Could you check a few things on this model? Use its own coordinates, in mm. Coordinates: 2 decimals unless noted, no trailing zeros. Write each loop counter-clockwise with the first axis right and the second up, starting at its lowest first coordinate (ties: lowest second). Pieces come first, ordered by that corner, then holes. Notation, with made-up numbers: M 48,81 L 99,81 A11 cw 99,93 Z; hole C 22.25,-25 d5. An arc over 180 degrees is marked long. Write item = value, one per line.
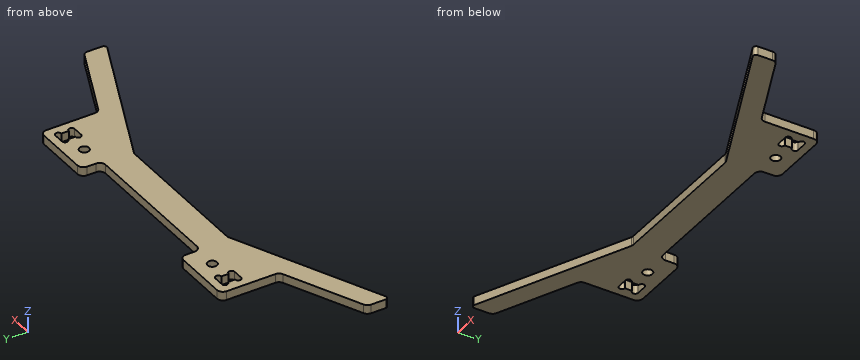
```python
from build123d import *

# Parameters (mm, degrees)
EXTRUDE_1_DEPTH     = 3
SKETCH_2_W          = 83.2
SKETCH_2_H          = 9
EXTRUDE_2_DEPTH     = 3
SKETCH_3_W          = 42.77133807
SKETCH_3_H          = 9.521513309
CUT_EXTRUDE_1_DEPTH = 3
EXTRUDE_3_DEPTH     = 3
CUT_EXTRUDE_2_DEPTH = 3
EXTRUDE_4_DEPTH     = 3
SKETCH_6_R          = 1.6
CUT_EXTRUDE_3_DEPTH = 3
SKETCH_8_W          = 53.2
SKETCH_8_H          = 7
CUT_EXTRUDE_4_DEPTH = 10
FILLET_2_R          = 2
FILLET_3_R          = 1


with BuildPart() as part:
    # 草图1 → 凸台-拉伸1 (new body)
    with BuildSketch(Plane.XY):
        Polygon((76.365250313, 0), (0, 34), (-76.365250313, 0), (-76.365250313, 6.567817671), (0, 40.567817671), (76.365250313, 6.567817671), align=None)
    extrude(amount=EXTRUDE_1_DEPTH)

    # 草图2 → 凸台-拉伸2 (add)
    with BuildSketch(Plane.XY.offset(3)):
        with Locations((0, 26.546304362)):
            Rectangle(SKETCH_2_W, SKETCH_2_H)
    extrude(amount=-EXTRUDE_2_DEPTH)

    # 草图3 → 切除-拉伸1 (cut)
    with BuildSketch(Plane.XY.offset(3)):
        with Locations((0, 35.807061017)):
            Rectangle(SKETCH_3_W, SKETCH_3_H)
    extrude(amount=-CUT_EXTRUDE_1_DEPTH, mode=Mode.SUBTRACT)

    # 草图4 → 凸台-拉伸3 (add)
    with BuildSketch(Plane.XY.offset(3)):
        Polygon((41.6, 31.046304362), (48.6, 31.046304362), (48.6, 18.929703565), (41.6, 22.046304362), align=None)
        Polygon((-41.6, 31.046304362), (-48.6, 31.046304362), (-48.6, 18.929703565), (-41.6, 22.046304362), align=None)
    extrude(amount=-EXTRUDE_3_DEPTH)

    # 草图5 → 切除-拉伸2 (cut)
    with BuildSketch(Plane.XY.offset(3)):
        with BuildLine():
            Line((-44.85, 28.296304362), (-41.35, 28.296304362))
            ThreePointArc((-41.35, 28.296304362), (-40.35, 27.296304362), (-41.35, 26.296304362))
            Line((-41.35, 26.296304362), (-41.35, 23.796304362))
            ThreePointArc((-41.35, 23.796304362), (-40.35, 22.796304362), (-41.35, 21.796304362))
            Line((-41.35, 21.796304362), (-44.85, 21.796304362))
            ThreePointArc((-44.85, 21.796304362), (-45.85, 22.796304362), (-44.85, 23.796304362))
            Line((-44.85, 23.796304362), (-44.85, 26.296304362))
            ThreePointArc((-44.85, 26.296304362), (-45.85, 27.296304362), (-44.85, 28.296304362))
        make_face()
        with BuildLine():
            Line((41.35, 26.296304362), (41.35, 23.796304362))
            ThreePointArc((41.35, 23.796304362), (40.35, 22.796304362), (41.35, 21.796304362))
            Line((41.35, 21.796304362), (44.85, 21.796304362))
            ThreePointArc((44.85, 21.796304362), (45.85, 22.796304362), (44.85, 23.796304362))
            Line((44.85, 23.796304362), (44.85, 26.296304362))
            ThreePointArc((44.85, 26.296304362), (45.85, 27.296304362), (44.85, 28.296304362))
            Line((44.85, 28.296304362), (41.35, 28.296304362))
            ThreePointArc((41.35, 28.296304362), (40.35, 27.296304362), (41.35, 26.296304362))
        make_face()
    extrude(amount=-CUT_EXTRUDE_2_DEPTH, mode=Mode.SUBTRACT)

    # 草图7 → 凸台-拉伸4 (add)
    with BuildSketch(Plane.XY.offset(3)):
        Polygon((26.848439987, 22.046304362), (76.365250313, 0), (76.365250313, -8.757090228), (25.147987493, 14.046304362), (-25.147987493, 14.046304362), (-76.365250313, -8.757090228), (-76.365250313, 0), (-26.848439987, 22.046304362), align=None)
    extrude(amount=-EXTRUDE_4_DEPTH)

    # 草图6 → 切除-拉伸3 (cut)
    with BuildSketch(Plane(origin=(0, 0, 0), x_dir=(-1, 0, 0), z_dir=(0, 0, -1))):
        with Locations((-34.5, 25.046304362)):
            Circle(SKETCH_6_R)
        with Locations(Location((34.5, 25.046304362, 0), (0, 0, 180))):
            Circle(SKETCH_6_R)
    extrude(amount=-CUT_EXTRUDE_3_DEPTH, mode=Mode.SUBTRACT)

    # 草图8 → 切除-拉伸4 (cut)
    with BuildSketch(Plane.XY.offset(3)):
        Polygon((-76.365250313, -1.094636279), (-48.6, 11.267249615), (-48.6, 18.929703565), (-76.365250313, 6.567817671), align=None)
        with Locations((0, 27.546304362)):
            Rectangle(SKETCH_8_W, SKETCH_8_H)
        Polygon((48.6, 18.929703565), (76.365250313, 6.567817671), (76.365250313, -1.094636279), (48.6, 11.267249615), align=None)
    extrude(amount=-CUT_EXTRUDE_4_DEPTH, mode=Mode.SUBTRACT)

    # 圆角2
    fillet_2_edges = [part.edges().sort_by_distance(p)[0] for p in [
        (25.147987493, 14.046304362, 1.5),
        (-25.147987493, 14.046304362, 1.5),
        (-26.6, 31.046304362, 1.5),
        (26.6, 31.046304362, 1.5),
        (-76.365250313, -1.094636279, 1.5),
        (-48.6, 11.267249615, 1.5),
        (26.6, 24.046304362, 1.5),
        (-26.6, 24.046304362, 1.5),
        (48.6, 11.267249615, 1.5),
        (76.365250313, -1.094636279, 1.5),
        (48.6, 31.046304362, 1.5),
        (-48.6, 31.046304362, 1.5),
    ]]
    fillet(fillet_2_edges, radius=FILLET_2_R)

    # 圆角3
    fillet_3_edges = [part.edges().sort_by_distance(p)[0] for p in [
        (76.365250313, -8.757090228, 1.5),
        (-76.365250313, -8.757090228, 1.5),
    ]]
    fillet(fillet_3_edges, radius=FILLET_3_R)


solid = part.part
```
Item 1: Imagine slicing it at D-D (x = -20). Write out the boundary of the cut face in (y, z), and give its area (3 significant figures).
Numbers:
outline = M 14.05,0 L 24.05,0 L 24.05,3 L 14.05,3 Z
area = 30.0 mm²
Item 2: If I drill on line 1 along X through (y, z) = (29, 1.45); line 2 along X through (y, z) = (18.5, 0.8); line 3 along X through (y, z) = (27, 1.3), over which ranges is the centre line in solid material (lowest first)?
Numbers:
line_1 = -48.6 to -26.6, 26.6 to 48.6
line_2 = -48.6 to 48.6
line_3 = -48.6 to -45.81, -40.39 to -26.6, 26.6 to 40.39, 45.81 to 48.6
Item 3: Imagine slicing it at B-B (y = -5). Write out the boundary of the cut face in (x, z), and give its area (3 significant figures).
Numbers:
outline = M -76.37,0 L -67.93,0 L -67.93,3 L -76.37,3 Z; M 67.93,0 L 76.37,0 L 76.37,3 L 67.93,3 Z
area = 50.6 mm²
Item 4: Imagine slicing it at C-C (y = 17.5). Write out the boundary of the cut face in (x, z), and give its area (3 significant figures).
Numbers:
outline = M -48.6,0 L 48.6,0 L 48.6,3 L -48.6,3 Z
area = 292 mm²
Item 5: I'm going to push flat-ended pins straight in: P1, Ø0.8, axis at y = 24.5, z = 1.5, coming from the -X side; P2, Ø1.2, axis at y = 24.5, z = 1, coming from the +X side; P3, Ø1, axis at x = 11.5, z = 1, coming from the +Y side. Where does each tip first touch, or does it pass through?
Numbers:
P1 = -48.6
P2 = 48.6
P3 = 24.05
Item 6: Imagine slicing it at A-A (x = 34.5). Write out the boundary of the cut face in (y, z).
Numbers:
outline = M 9.88,0 L 23.45,0 L 23.45,3 L 9.88,3 Z; M 26.65,0 L 31.05,0 L 31.05,3 L 26.65,3 Z
